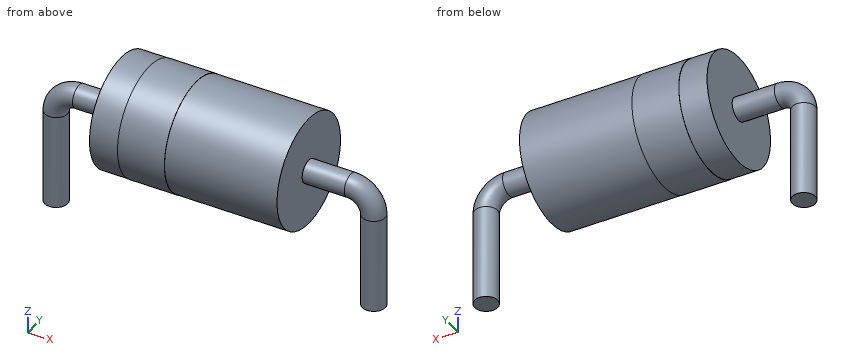
from build123d import *

# Parameters (mm, degrees)
SKETCH002_W = 9
SKETCH002_H = 2.65
SKETCH_R    = 0.55
SKETCH003_W = 2.25
SKETCH003_H = 0.02


with BuildPart() as revolution:
    # Sketch002 → Revolution (revolve)
    with BuildSketch(Plane.XZ):
        with Locations((7.62, 4.475)):
            Rectangle(SKETCH002_W, SKETCH002_H)
    revolve(axis=Axis((3.12, 0, 3.15), (1, 0, 0)))


with BuildPart() as sweep_body:
    # Sweep: sweep along a path in Sketch001
    with BuildLine(Plane.XZ) as sweep_path:
        Line((0, -2.5), (0, 2.05))
        ThreePointArc((0, 2.05), (0.322183, 2.827817), (1.1, 3.15))
        Line((1.1, 3.15), (14.14, 3.15))
        ThreePointArc((14.14, 3.15), (14.917817, 2.827817), (15.24, 2.05))
        Line((15.24, 2.05), (15.24, -2.5))
    # Sketch → Sweep (sweep)
    with BuildSketch(Plane.XY.offset(-2)):
        Circle(SKETCH_R)
    sweep(path=sweep_path.line)


with BuildPart() as obj1:
    # Sketch003 → Revolution001 (revolve)
    with BuildSketch(Plane.XZ):
        with Locations((5.595, 5.8)):
            Rectangle(SKETCH003_W, SKETCH003_H)
    revolve(axis=Axis((0, 0, 3.15), (1, 0, 0)))

    add(revolution.part)
    add(sweep_body.part)


solid = obj1.part
The listing builds one solid part. Answer for the finished solid, in the listing's coordinates (mm). Coordinates: 2 decimals unless noted, no trailing zeros. Loops run counter-clockwise (first coordinate to the right, second up) from the corner with the lowest first, then second, coordinate; pieces in that order, holes last. Notation, with made-up numbers: M 59,-12 L 97,-12 A21 cw 97,18 Z; hole C -31.5,0.5 d11. An arc over 180 degrees is marked long. Answer in a Markdown table with one row per item.
1) Find section D-D (z = 1.25). Count the separate pieces of the cut face and the enclosed holes in it, then the cut area to 3 significant figures.
Answers below:
| item | result |
|---|---|
| separate pieces | 3 |
| enclosed holes | 0 |
| area | 35.2 mm^2 |
2) Find section C-C (x = 6). Determine the outline of the cut face in (y, z).
Answers below:
| item | result |
|---|---|
| outline | C 0,3.15 d5.32 |
3) Find the intervals of material crossed by probe 1 along X at (y, z) = (0.2, 1); probe 2 along X at (y, z) = (0.7, 4.25); probe 3 along Z at (x, y) = (9.75, 0.15), in increasing order.
Answers below:
| item | result |
|---|---|
| probe 1 | -0.51 to 0.51, 3.12 to 12.12, 14.73 to 15.75 |
| probe 2 | 3.12 to 12.12 |
| probe 3 | 0.5 to 5.8 |
4) Given pin 1 (2 mm diameter, centred on x = 7, z = 3, fed in from +Y), flat-ended and moving along its own axis, determine where the tip first touches the part or whether it passes through.
Answers below:
| item | result |
|---|---|
| pin 1 | y = 2.66 |
